Part model, mm, in its own coordinate system. A direction names the side the tool comes from. Give positions to 0.01 mm unless a question says otherwise; leave off trailing zeros. Write each loop counter-clockwise with the first axis right and the second up, starting at its lowest first coordinate (ties: lowest second). Pieces come first, ordered by that corner, then holes.
```python
from build123d import *

# Parameters (mm, degrees)
BASE_FLANGE1_DEPTH            = 1.1
EDGE_FLANGE1_STRIP_W          = 5.8732
EDGE_FLANGE1_STRIP_H          = 1.1
EDGE_FLANGE1_STRIP_CUT_DEPTH  = 9.1
EDGE_FLANGE1_RELIEF_W         = 6.4232
EDGE_FLANGE1_RELIEF_H         = 0.55
EDGE_FLANGE1_RELIEF_CUT_DEPTH = 1.1
EDGE_FLANGE1_DEPTH            = 9.1
EDGE_FLANGE2_STRIP_W          = 5.8732
EDGE_FLANGE2_STRIP_H          = 1.1
EDGE_FLANGE2_STRIP_CUT_DEPTH  = 9.1
EDGE_FLANGE2_DEPTH            = 9.1
SKETCH9_R                     = 1.65
EXTRUDE1_DEPTH                = 1.1
SKETCHED_START                = -55.937504649
SKETCHED_BEND2_DEPTH          = 84.037504649
SKETCHED_START_2              = -37.556301802
SKETCHED_BEND2_2_OUTLINE_W    = 35.581961475
SKETCHED_BEND2_2_OUTLINE_H    = 1.1
SKETCHED_BEND2_2_DEPTH        = 32.156301802
SKETCHED_START_3              = -20
SKETCHED_BEND2_3_DEPTH        = 14.6
SKETCHED_START_4              = 19.2
SKETCHED_BEND2_4_DEPTH        = 8.9
SKETCHED_START_5              = -19.700000012
SKETCHED_BEND2_5_DEPTH        = 1.100000011
SKETCHED_BEND5_DEPTH          = 84.037504649
SKETCHED_BEND5_2_OUTLINE_W    = 1.1
SKETCHED_BEND5_2_OUTLINE_H    = 35.581961474
SKETCHED_BEND5_2_DEPTH        = 32.156301802
SKETCHED_BEND5_3_DEPTH        = 14.6
SKETCHED_BEND5_4_DEPTH        = 8.9
SKETCHED_START_6              = 10.352213433
SKETCHED_BEND5_5_DEPTH        = 1.1


with BuildPart() as part:
    # Base-Flange1: sheet metal written as solids
    # Sketch1 → Base-Flange1 (new body)
    with BuildSketch(Plane(origin=(0, 0, 0), x_dir=(1, 0, 0), z_dir=(0, 1, 0))):
        with BuildLine():
            Line((-30.1, 1.2), (-21, 1.2))
            Line((-21, 1.2), (-21, -0.6))
            Line((-21, -0.6), (-20, -0.6))
            Line((-20, -0.6), (-20, 19.7))
            Line((-20, 19.7), (-20, 32.054788892))
            Line((-20, 32.054788892), (-20, 35.211930536))
            Line((-20, 35.211930536), (-55.937504649, 35.211930536))
            Line((-55.937504649, 35.211930536), (-55.937504649, 52.412689164))
            Line((-55.937504649, 52.412689164), (-37.556301802, 70.793892011))
            Line((-37.556301802, 70.793892011), (-1.637070551, 70.793892011))
            Line((-1.637070551, 70.793892011), (28.1, 39.427802749))
            Line((28.1, 39.427802749), (28.1, 32.054788892))
            Line((28.1, 32.054788892), (28.1, 19.7))
            Line((28.1, 19.7), (28.1, -4.05))
            ThreePointArc((28.1, -4.05), (26.928427125, -6.878427125), (24.1, -8.05))
            Line((24.1, -8.05), (18.1, -8.05))
            ThreePointArc((18.1, -8.05), (14.863529932, -15.863529932), (7.05, -19.1))
            Line((7.05, -19.1), (-10.1, -19.1))
            ThreePointArc((-10.1, -19.1), (-16.605382387, -16.405382387), (-19.3, -9.9))
            Line((-19.3, -9.9), (-26.1, -9.9))
            ThreePointArc((-26.1, -9.9), (-28.928427125, -8.728427125), (-30.1, -5.9))
            Line((-30.1, -5.9), (-30.1, 1.2))
        make_face()
        with BuildLine():
            Line((-5.4, 19.7), (-5.4, 16.8))
            Line((-5.4, 16.8), (19.2, 16.8))
            Line((19.2, 16.8), (19.2, 19.7))
            Line((19.2, 19.7), (19.2, 32.054788892))
            ThreePointArc((19.2, 32.054788892), (6.9, 44.354788892), (-5.4, 32.054788892))
            Line((-5.4, 32.054788892), (-5.4, 19.7))
        make_face(mode=Mode.SUBTRACT)
    extrude(amount=BASE_FLANGE1_DEPTH)

    # Edge-Flange1: sheet metal written as solids
    # Edge-Flange1 strip (on a plane across the edge) → Edge-Flange1 strip cut (cut)
    with BuildSketch(Plane(origin=(-21, 1.1, -1.2), x_dir=(0, 0, 1), z_dir=(-1, 0, 0))):
        with Locations((-1.1, -0.55)):
            Rectangle(EDGE_FLANGE1_STRIP_W, EDGE_FLANGE1_STRIP_H)
    extrude(amount=EDGE_FLANGE1_STRIP_CUT_DEPTH, mode=Mode.SUBTRACT)

    # Edge-Flange1 relief (on the sheet) → Edge-Flange1 relief cut (cut)
    with BuildSketch(Plane(origin=(-21, 1.1, 0.6366), x_dir=(0, 0, 1), z_dir=(0, 1, 0))):
        with Locations((-2.6616, 0.275)):
            Rectangle(EDGE_FLANGE1_RELIEF_W, EDGE_FLANGE1_RELIEF_H)
    extrude(amount=-EDGE_FLANGE1_RELIEF_CUT_DEPTH, mode=Mode.SUBTRACT)

    # Edge-Flange1 section (on a plane across the edge) → Edge-Flange1 (add)
    with BuildSketch(Plane(origin=(-21, 1.1, -1.2), x_dir=(0, 0, 1), z_dir=(-1, 0, 0))):
        with BuildLine():
            Line((0, 0.7366), (0, 5.8))
            Line((0, 5.8), (1.1, 5.8))
            Line((1.1, 5.8), (1.1, 0.7366))
            ThreePointArc((1.1, 0.7366), (1.315745145, 0.215745145), (1.8366, 0))
            Line((1.8366, 0), (1.8366, -1.1))
            ThreePointArc((1.8366, -1.1), (0.537927686, -0.562072314), (0, 0.7366))
        make_face()
    extrude(amount=EDGE_FLANGE1_DEPTH)

    # Edge-Flange2: sheet metal written as solids
    # Edge-Flange2 strip (on a plane across the edge) → Edge-Flange2 strip cut (cut)
    with BuildSketch(Plane(origin=(-30.1, 6.9, -1.2), x_dir=(0, -1, 0), z_dir=(1, 0, 0))):
        with Locations((-1.1, -0.55)):
            Rectangle(EDGE_FLANGE2_STRIP_W, EDGE_FLANGE2_STRIP_H)
    extrude(amount=EDGE_FLANGE2_STRIP_CUT_DEPTH, mode=Mode.SUBTRACT)

    # Edge-Flange2 section (on a plane across the edge) → Edge-Flange2 (add)
    with BuildSketch(Plane(origin=(-30.1, 6.9, -1.2), x_dir=(0, -1, 0), z_dir=(1, 0, 0))):
        with BuildLine():
            Line((0, 0.7366), (0, 8.2))
            Line((0, 8.2), (1.1, 8.2))
            Line((1.1, 8.2), (1.1, 0.7366))
            ThreePointArc((1.1, 0.7366), (1.315745145, 0.215745145), (1.8366, 0))
            Line((1.8366, 0), (1.8366, -1.1))
            ThreePointArc((1.8366, -1.1), (0.537927686, -0.562072314), (0, 0.7366))
        make_face()
    extrude(amount=EDGE_FLANGE2_DEPTH)

    # Sketch9 → Extrude1 (cut)
    with BuildSketch(Plane(origin=(0, 6.9, 0), x_dir=(1, 0, 0), z_dir=(0, 1, 0))):
        with Locations(Location((-25.55, 6.05, 0), (0, 0, 270))):
            Circle(SKETCH9_R)
        with BuildLine():
            Line((-30.1, 6.4), (-30.1, 9.4))
            Line((-30.1, 9.4), (-27.1, 9.4))
            ThreePointArc((-27.1, 9.4), (-29.221320344, 8.521320344), (-30.1, 6.4))
        make_face()
        with BuildLine():
            Line((-24, 9.4), (-21, 9.4))
            Line((-21, 9.4), (-21, 6.4))
            ThreePointArc((-21, 6.4), (-21.878679656, 8.521320344), (-24, 9.4))
        make_face()
    extrude(amount=-EXTRUDE1_DEPTH, mode=Mode.SUBTRACT)

    # Sketched Bend2: read off the stored shape, not the designer's step
    # Sketched Bend2 outline → Sketched Bend2 (cut)
    with BuildSketch(Plane.YZ.offset(SKETCHED_START)):
        with BuildLine():
            ThreePointArc((1.1, -19.545814945), (0.299404636, -18.868452246), (-1.3e-08, -17.8634))
            Line((-1.3e-08, -17.8634), (0, -70.793892011))
            Line((0, -70.793892011), (1.1, -70.793892011))
            Line((1.1, -70.793892011), (1.1, -19.545814945))
        make_face()
    extrude(amount=SKETCHED_BEND2_DEPTH, mode=Mode.SUBTRACT)



with BuildPart() as body_2:
    # Sketched Bend2 2 outline → Sketched Bend2 2 (new body)
    with BuildSketch(Plane.YZ.offset(SKETCHED_START_2)):
        with Locations((34.95512472, -19.15)):
            Rectangle(SKETCHED_BEND2_2_OUTLINE_W, SKETCHED_BEND2_2_OUTLINE_H)
    extrude(amount=SKETCHED_BEND2_2_DEPTH)


with BuildPart() as part_1:
    add(part.part)

    add(body_2.part)  # Sketched Bend2 3 merges body 2
    # Sketched Bend2 3 outline → Sketched Bend2 3 (add)
    with BuildSketch(Plane.YZ.offset(SKETCHED_START_3)):
        with BuildLine():
            Line((17.164143982, -18.6), (1.836600013, -18.600000013))
            ThreePointArc((1.836600013, -18.600000013), (1.315745141, -18.384254868), (1.099999987, -17.8634))
            Line((1.099999987, -17.8634), (1.1, -19.545814945))
            ThreePointArc((1.1, -19.545814945), (1.460317993, -19.661040525), (1.8366, -19.700000013))
            Line((1.8366, -19.700000013), (17.164143982, -19.7))
            Line((17.164143982, -19.7), (17.164143982, -18.6))
        make_face()
    extrude(amount=SKETCHED_BEND2_3_DEPTH)

    # Sketched Bend2 4 outline → Sketched Bend2 4 (add)
    with BuildSketch(Plane.YZ.offset(SKETCHED_START_4)):
        with BuildLine():
            Line((17.164143982, -18.6), (1.836600013, -18.600000013))
            ThreePointArc((1.836600013, -18.600000013), (1.315745141, -18.384254868), (1.099999987, -17.8634))
            Line((1.099999987, -17.8634), (1.1, -19.545814945))
            ThreePointArc((1.1, -19.545814945), (1.460317993, -19.661040525), (1.8366, -19.700000013))
            Line((1.8366, -19.700000013), (17.164143982, -19.7))
            Line((17.164143982, -19.7), (17.164143982, -18.6))
        make_face()
    extrude(amount=SKETCHED_BEND2_4_DEPTH)

    # Sketched Bend2 5 outline → Sketched Bend2 5 (add)
    with BuildSketch(Plane.XY.offset(SKETCHED_START_5)):
        Polygon((-37.556301802, 17.164143982), (-37.556301802, 52.746105457), (-55.937504649, 34.36490261), (-55.937504649, 17.164143982), align=None)
        with BuildLine():
            Line((28.1, 17.164143982), (28.1, 21.380016195))
            Line((28.1, 21.380016195), (-1.637070551, 52.746105457))
            Line((-1.637070551, 52.746105457), (-5.4, 52.746105457))
            Line((-5.4, 52.746105457), (-5.4, 14.007002338))
            ThreePointArc((-5.4, 14.007002338), (6.9, 26.307002338), (19.2, 14.007002338))
            Line((19.2, 14.007002338), (19.2, 17.164143982))
            Line((19.2, 17.164143982), (28.1, 17.164143982))
        make_face()
    extrude(amount=SKETCHED_BEND2_5_DEPTH)

    # Sketched Bend5: read off the stored shape, not the designer's step
    # Sketched Bend5 outline → Sketched Bend5 (cut)
    with BuildSketch(Plane.YZ.offset(SKETCHED_START)):
        with BuildLine():
            ThreePointArc((9.615613433, -18.599999993), (10.620665676, -18.89940464), (11.298028372, -19.7))
            Line((11.298028372, -19.7), (52.746105457, -19.7))
            Line((52.746105457, -19.7), (52.746105457, -18.6))
            Line((52.746105457, -18.6), (9.615613433, -18.599999993))
        make_face()
    extrude(amount=SKETCHED_BEND5_DEPTH, mode=Mode.SUBTRACT)



with BuildPart() as body_2_2:
    # Sketched Bend5 2 outline → Sketched Bend5 2 (new body)
    with BuildSketch(Plane.YZ.offset(SKETCHED_START_2)):
        with Locations((10.902213433, -43.755124732)):
            Rectangle(SKETCHED_BEND5_2_OUTLINE_W, SKETCHED_BEND5_2_OUTLINE_H)
    extrude(amount=SKETCHED_BEND5_2_DEPTH)


with BuildPart() as part_2:
    add(part_1.part)

    add(body_2_2.part)  # Sketched Bend5 3 merges body 2 2
    # Sketched Bend5 3 outline → Sketched Bend5 3 (add)
    with BuildSketch(Plane.YZ.offset(SKETCHED_START_3)):
        with BuildLine():
            ThreePointArc((11.45221344, -20.4366), (11.413253953, -20.060317993), (11.298028372, -19.7))
            Line((11.298028372, -19.7), (9.615613433, -19.699999993))
            ThreePointArc((9.615613433, -19.699999993), (10.136468293, -19.91574514), (10.35221344, -20.4366))
            Line((10.35221344, -20.4366), (10.352213433, -25.964143995))
            Line((10.352213433, -25.964143995), (11.452213433, -25.964143995))
            Line((11.452213433, -25.964143995), (11.45221344, -20.4366))
        make_face()
    extrude(amount=SKETCHED_BEND5_3_DEPTH)

    # Sketched Bend5 4 outline → Sketched Bend5 4 (add)
    with BuildSketch(Plane.YZ.offset(SKETCHED_START_4)):
        with BuildLine():
            ThreePointArc((11.45221344, -20.4366), (11.413253953, -20.060317993), (11.298028372, -19.7))
            Line((11.298028372, -19.7), (9.615613433, -19.699999993))
            ThreePointArc((9.615613433, -19.699999993), (10.136468293, -19.91574514), (10.35221344, -20.4366))
            Line((10.35221344, -20.4366), (10.352213433, -25.964143995))
            Line((10.352213433, -25.964143995), (11.452213433, -25.964143995))
            Line((11.452213433, -25.964143995), (11.45221344, -20.4366))
        make_face()
    extrude(amount=SKETCHED_BEND5_4_DEPTH)

    # Sketched Bend5 5 outline → Sketched Bend5 5 (add)
    with BuildSketch(Plane(origin=(0, 0, 0), x_dir=(1, 0, 0), z_dir=(0, 1, 0)).offset(SKETCHED_START_6)):
        Polygon((-37.556301802, 25.964143995), (-37.556301802, 61.546105469), (-55.937504649, 43.164902622), (-55.937504649, 25.964143995), align=None)
        with BuildLine():
            Line((28.1, 25.964143995), (28.1, 30.180016207))
            Line((28.1, 30.180016207), (-1.637070551, 61.546105469))
            Line((-1.637070551, 61.546105469), (-5.4, 61.546105469))
            Line((-5.4, 61.546105469), (-5.4, 22.80700235))
            ThreePointArc((-5.4, 22.80700235), (6.9, 35.10700235), (19.2, 22.80700235))
            Line((19.2, 22.80700235), (19.2, 25.964143995))
            Line((19.2, 25.964143995), (28.1, 25.964143995))
        make_face()
    extrude(amount=SKETCHED_BEND5_5_DEPTH)


solid = part_2.part
```
1) Pin check, flat tips, straight feed: pin 1 Ø10 at (x, z) = (10.5, -46.5) entering from -Y; pin 2 Ø0.6 at (x, y) = (10.5, 0.5) entering from -Z; pin 3 Ø1.6 at (x, y) = (-25.5, 3.5) entering from +Z; pin 4 Ø1.8 at (y, z) = (5, -20.5) entering from +X. Stop position of each tip, or through.
Answers follow:
pin 1: stops at y = 10.35
pin 2: stops at z = -16.8
pin 3: stops at z = -0.1
pin 4: stops at x = 28.1
2) Two-plate mould, pull along Z, no slides. Class faces 1 (the face through (-27.16, 6.36, -6.41)), 2 (the face through (-28.897, 0.542, 8.759)), 3 (the face through (-1, 1.1, 0)): +Z half, -Z half, draft (parallel to the pull), parting line (faces both ways), or undercut.
Answers follow:
face 1: undercut
face 2: +Z half
face 3: draft
3) 3-axis set-ups, long thin cutter, end or side, ignore diameter. For faces 4 (the face through (-26, 6.9, -4)), 5 (the face through (-21.86, 6.36, -8.5)), 6 (the face through (-21, 4, -1)), 7 (the face through (24, 6, -19.7)), 8 (the face through (24, 6, -18.6)): which of +Z, -Z, +X, -X, +Y, -Y reach the whole face in a straight line?
Answers follow:
face 4: +Z, -Z, +X, -X, +Y
face 5: -Z, +X, +Y, -Y
face 6: -Z, +Y, -Y
face 7: -Z, +X, -X, -Y
face 8: +Z, +X, -X, +Y
4) Saw through at A-A, the plane x = 13. Write the cut outline in (y, z), then the cut area to 3 significant figures.
Answers follow:
outline: (0, -16.8) - (1.1, -16.8) - (1.1, 17.36) - (0, 17.36) - close; (10.35, -46.11) - (11.45, -46.11) - (11.45, -33.49) - (10.35, -33.49) - close
area: 51.5 mm2
5) Wall check: L1, parallel to X at y = 6.6, z = -6.05; L2, parallel to Z at x = 21, y = 4.5; L3, parallel to Z at x = -23.5, y = 2. Give the ranges that are in metal, low to high.
Answers follow:
L1: x = -30.1 to -27.2, -23.9 to -21
L2: z = -19.7 to -18.6
L3: z = -1.2 to -0.1
6) Saw through at C-C, the plane x = -35. Write the cut outline in (y, z).
Answers follow:
outline: (10.35, -61.55) - (11.45, -61.55) - (11.45, -25.96) - (10.35, -25.96) - close
7) Saw through at B-B, the plane x = -7. Write the cut outline in (y, z).
Answers follow:
outline: (0, -17.86) arc R1.84 ccw to (1.84, -19.7) - (9.62, -19.7) arc R0.74 cw to (10.35, -20.44) - (10.35, -61.55) - (11.45, -61.55) - (11.45, -20.44) arc R1.84 ccw to (9.62, -18.6) - (1.84, -18.6) arc R0.74 cw to (1.1, -17.86) - (1.1, 19.1) - (0, 19.1) - close
